Part print with two shaded views. Sizes in mm from the minimum x, y, z corner. A direction names the side the tool comes from. Coordinates: 2 decimals unless noted, no trailing zeros. Loops run counter-clockwise (first coordinate to the right, second up) from the corner with the lowest first, then second, coordinate; pieces in that order, holes last.
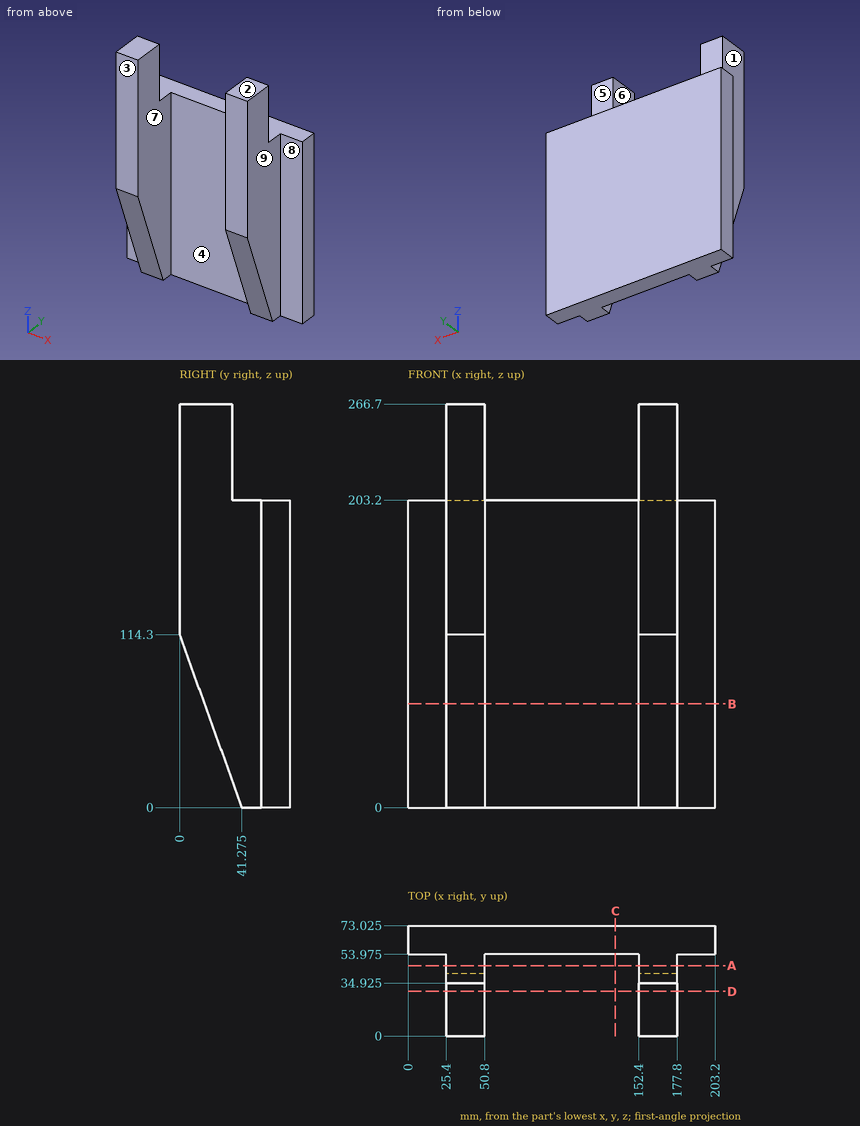
Q1. Mould opens along X. For the marked faces 6, 7, 8 and 9 say: +X half, -X half, draft (parallel to the pull), parting line (faces both ways), or undercut.
Answers:
face 6: undercut
face 7: undercut
face 8: draft
face 9: +X half
Q2. Slice it at C-C (x = 137). List the corners of the cut face in (y, z) (3 decimals), and give its area (3 significant figures).
Answers:
outline: (53.975, 0) - (73.025, 0) - (73.025, 203.2) - (53.975, 203.2) - close
area: 3,870 mm2
Q3. Slice it at D-D (y = 29.5). List the corners of the cut face in (x, z).
Answers:
outline: (25.4, 32.61) - (50.8, 32.61) - (50.8, 266.7) - (25.4, 266.7) - close; (152.4, 32.61) - (177.8, 32.61) - (177.8, 266.7) - (152.4, 266.7) - close
Q4. Slice it at A-A (y = 46.5). List the corners of the cut face in (x, z), and give its area (3 significant figures).
Answers:
outline: (25.4, 0) - (50.8, 0) - (50.8, 203.2) - (25.4, 203.2) - close; (152.4, 0) - (177.8, 0) - (177.8, 203.2) - (152.4, 203.2) - close
area: 10,300 mm2
Q5. Which spindle directions (+Z, -Z, +X, -X, +Y, -Y) get a long thin tool onto all of the face, cutting with end or side? Do the marked faces 1, 2, 3, 4 and 5. Say none if no direction does.
Answers:
face 1: +Z, -Z, -X, -Y
face 2: +Z, +X, -X, +Y, -Y
face 3: +Z, -Z, +X, -X, -Y
face 4: +Z, -Z, -Y
face 5: +Z, +X, -X, +Y
Q6. Flat gauge pins, fed straight in: P1, Ø20.5, axis at x = 192, z = 112.5, coming from the -Y side (3 decimals); P2, Ø5, axis at y = 20.5, z = 218.5, coming from the +X side; P3, Ø20.5, axis at x = 170.5, z = 220.5, coming from the +Y side (3 decimals). Where does each tip first touch, or does it go through?
Answers:
P1: stops at y = 53.975
P2: stops at x = 177.8
P3: stops at y = 34.925
Q7. Slice it at B-B (z = 68.5). List the corners of the cut face in (x, y) (3 decimals), and give its area (3 significant figures).
Answers:
outline: (0, 53.975) - (25.4, 53.975) - (25.4, 16.539) - (50.8, 16.539) - (50.8, 53.975) - (152.4, 53.975) - (152.4, 16.539) - (177.8, 16.539) - (177.8, 53.975) - (203.2, 53.975) - (203.2, 73.025) - (0, 73.025) - close
area: 5,770 mm2
Q8. Drill centre lines: line 1 (X direction, y = 30, z = 222.5); line 2 (Y direction, x = 79.5, z = 101.5) (3 decimals); line 3 (Z direction, x = 173.5, y = 59). Where is each one in solid material? Low to high.
Answers:
line 1: x = 25.4 to 50.8, 152.4 to 177.8
line 2: y = 53.975 to 73.025
line 3: z = 0 to 203.2
